```python
from build123d import *

# Parameters (mm, degrees)
SKETCH_1_W          = 100
SKETCH_1_H          = 154
SKETCH_1_R          = 2.5
EXTRUDE_1_DEPTH     = 3
SKETCH_4_R          = 1.25
CUT_EXTRUDE_1_DEPTH = 3
CUT_EXTRUDE_2_DEPTH = 10
CUT_EXTRUDE_3_DEPTH = 10


with BuildPart() as part:
    # 스케치1 → 보스-돌출1 (new body)
    with BuildSketch(Plane(origin=(0, -15.691888839, 0), x_dir=(1, 0, 0), z_dir=(0, 1, 0))):
        with Locations((994.328, -155.973817188)):
            Rectangle(SKETCH_1_W, SKETCH_1_H)
        with Locations(Location((1034.328, -88.973817188, 0), (0, 0, 270))):
            Circle(SKETCH_1_R, mode=Mode.SUBTRACT)
        with Locations(Location((1034.328, -222.973817188, 0), (0, 0, 270))):
            Circle(SKETCH_1_R, mode=Mode.SUBTRACT)
        with Locations(Location((954.328, -223.956502664, 0), (0, 0, 270))):
            Circle(SKETCH_1_R, mode=Mode.SUBTRACT)
        with Locations(Location((954.328, -88.973817188, 0), (0, 0, 270))):
            Circle(SKETCH_1_R, mode=Mode.SUBTRACT)
    extrude(amount=EXTRUDE_1_DEPTH)

    # 스케치4 → 컷-돌출1 (cut)
    with BuildSketch(Plane(origin=(0, -12.691888839, 0), x_dir=(1, 0, 0), z_dir=(0, 1, 0))):
        with Locations(Location((969.801034838, -137.973817188, 0), (0, 0, 270))):
            Circle(SKETCH_4_R)
        with Locations(Location((1005.801034838, -137.973817188, 0), (0, 0, 270))):
            Circle(SKETCH_4_R)
        with Locations(Location((1005.801034838, -173.973817188, 0), (0, 0, 270))):
            Circle(SKETCH_4_R)
        with Locations(Location((969.801034838, -173.973817188, 0), (0, 0, 270))):
            Circle(SKETCH_4_R)
        with Locations(Location((993.801034838, -137.973817188, 0), (0, 0, 270))):
            Circle(SKETCH_4_R)
        with Locations(Location((981.801034838, -137.973817188, 0), (0, 0, 270))):
            Circle(SKETCH_4_R)
        with Locations(Location((981.801034838, -173.973817188, 0), (0, 0, 270))):
            Circle(SKETCH_4_R)
        with Locations(Location((993.801034838, -173.973817188, 0), (0, 0, 270))):
            Circle(SKETCH_4_R)
    extrude(amount=-CUT_EXTRUDE_1_DEPTH, mode=Mode.SUBTRACT)

    # 스케치5 → 컷-돌출2 (cut)
    with BuildSketch(Plane(origin=(0, -12.691888839, 0), x_dir=(1, 0, 0), z_dir=(0, 1, 0))):
        with BuildLine():
            Line((964.328, -78.875628165), (1024.328, -78.875628165))
            Line((1024.328, -78.875628165), (1024.328, -113.973817188))
            ThreePointArc((1024.328, -113.973817188), (1021.399067812, -121.044884999), (1014.328, -123.973817188))
            Line((1014.328, -123.973817188), (974.328, -123.973817188))
            ThreePointArc((974.328, -123.973817188), (967.256932188, -121.044884999), (964.328, -113.973817188))
            Line((964.328, -113.973817188), (964.328, -78.875628165))
        make_face()
        with BuildLine():
            Line((964.328, -238.398898185), (1024.328, -238.398898185))
            Line((1024.328, -238.398898185), (1024.328, -197.973817188))
            ThreePointArc((1024.328, -197.973817188), (1021.399067812, -190.902749376), (1014.328, -187.973817188))
            Line((1014.328, -187.973817188), (974.328, -187.973817188))
            ThreePointArc((974.328, -187.973817188), (967.256932188, -190.902749376), (964.328, -197.973817188))
            Line((964.328, -197.973817188), (964.328, -238.398898185))
        make_face()
    extrude(amount=-CUT_EXTRUDE_2_DEPTH, mode=Mode.SUBTRACT)

    # 스케치6 → 컷-돌출3 (cut)
    with BuildSketch(Plane(origin=(0, -12.691888839, 0), x_dir=(1, 0, 0), z_dir=(0, 1, 0))):
        with BuildLine():
            Line((964.328, -145.973817188), (1024.328, -145.973817188))
            ThreePointArc((1024.328, -145.973817188), (1034.328, -155.973817188), (1024.328, -165.973817188))
            Line((1024.328, -165.973817188), (964.328, -165.973817188))
            ThreePointArc((964.328, -165.973817188), (954.328, -155.973817188), (964.328, -145.973817188))
        make_face()
    extrude(amount=-CUT_EXTRUDE_3_DEPTH, mode=Mode.SUBTRACT)


solid = part.part
```
Model file for the job. Use its own axes, mm. A direction names the side the tool comes from. Round coordinates to 2 decimals unless told otherwise and drop trailing zeros. Write each loop counter-clockwise with the first axis right and the second up, starting at its lowest first coordinate (ties: lowest second). Pieces come first, ordered by that corner, then holes. Notation, with made-up numbers: (-24.75, -19) - (25.25, -19) arc R21 cw to (25.25, 7) - close; hole circle Ø2 at (32, -14). An arc over 180 degrees is marked (long way). One line per item, written item: value.
(1) Cut at C-C, the plane z = 223. Give the cut face in (x, y), plus the area to 3 significant figures.
Values follow:
outline: (944.33, -15.69) - (952.02, -15.69) - (952.02, -12.69) - (944.33, -12.69) - close; (956.64, -15.69) - (964.33, -15.69) - (964.33, -12.69) - (956.64, -12.69) - close; (1024.33, -15.69) - (1031.83, -15.69) - (1031.83, -12.69) - (1024.33, -12.69) - close; (1036.83, -15.69) - (1044.33, -15.69) - (1044.33, -12.69) - (1036.83, -12.69) - close
area: 91.1 mm²
(2) Two-plate mould, pull along Z, no slides. Class faces 1 (the flat face through (954, -14, 78.974)), 2 (the cylindrical face through (1031.887, -14.213, 222.432)), 3 (the flat face through (1044.328, -14, 157)): pulls with the +Z half, pulls with the -Z half, needs draft (parallel to the pull), parting line crosses it, or undercut.
Values follow:
face 1: pulls with the -Z half
face 2: undercut
face 3: needs draft
(3) 3-axis set-ups, long thin cutter, end or side, ignore diameter. For faces 4 (the cylindrical face through (1021.476, -14.171, 190.981)), 5 (the cylindrical face through (1021.476, -14.171, 120.967)), 6 (the flat face through (994, -14, 145.974)), 7 (the flat face through (1034, -14, 232.974)): which of +Z, -Z, +X, -X, +Y, -Y reach the whole face in a straight line?
Values follow:
face 4: +Z, +Y, -Y
face 5: -Z, +Y, -Y
face 6: +Y, -Y
face 7: +Z, +X, -X, +Y, -Y
(4) Cut at D-D, the plane y = -15. Give the number of separate pieces and of enclosed holes in the cut face, plus the area to 3 significant figures.
Values follow:
separate pieces: 1
enclosed holes: 13
area: 8,450 mm²
(5) Wall check: probe 1 along Z at (x, y) = (988.5, -14.4); probe 2 along X at (y, z) = (-13.55, 100); probe 3 along Z at (x, y) = (953.5, -14.25). Give the ranges that are in metal, low to high.
Values follow:
probe 1: z = 123.97 to 145.97, 165.97 to 187.97
probe 2: x = 944.33 to 964.33, 1024.33 to 1044.33
probe 3: z = 78.97 to 86.61, 91.33 to 221.6, 226.32 to 232.97
(6) Cut at B-B, the plane z = 95. Give the cut face in (x, y).
Values follow:
outline: (944.33, -15.69) - (964.33, -15.69) - (964.33, -12.69) - (944.33, -12.69) - close; (1024.33, -15.69) - (1044.33, -15.69) - (1044.33, -12.69) - (1024.33, -12.69) - close
(7) Drop flat-ended pins along their axis: P1, Ø3, axis at x = 981.8, z = 137.97, coming from the -Y side; P2, Ø0.9, axis at x = 986, y = -14, coming from the -Z side; P3, Ø1.5, axis at x = 969.8, z = 173.97, coming from the -Y side; P4, Ø1.5, axis at x = 990.5, y = -15, coming from the +Z side. Give the stop position or say it passes through.
Values follow:
P1: stops at y = -15.69
P2: stops at z = 123.97
P3: passes through
P4: stops at z = 187.97
(8) Cut at A-A, the plane x = 1001.5. Give the cut face in (y, z).
Values follow:
outline: (-15.69, 123.97) - (-12.69, 123.97) - (-12.69, 145.97) - (-15.69, 145.97) - close; (-15.69, 165.97) - (-12.69, 165.97) - (-12.69, 187.97) - (-15.69, 187.97) - close
